Build history of the part. All positions in model axes, mm. A direction names the side the tool comes from. Give positions to 0.01 mm unless a question says otherwise; leave off trailing zeros. Loops run counter-clockwise (first coordinate to the right, second up) from the corner with the lowest first, then second, coordinate; pieces in that order, holes last. Notation, with made-up numbers: (49, 69.25) -> (99, 69.25) arc R20 ccw to (99, 95.25) -> close; hole circle Ø1 at (5, -6). An arc over 180 degrees is marked (long way). Answer in a Markdown table with one row per item. Add a question column.
from build123d import *

# Parameters (mm, degrees)
F1_DEPTH = 76.2
F2_R     = 38.1


# Not quite as in the source:
# - ends of sketch curves that miss each other by under 0.0002 mm in the source are joined


with BuildPart() as f1:
    # F0 (on Top) → F1 (new body, symmetric)
    with BuildSketch(Plane.XY):
        Polygon((21.6444802228, 76.2), (-21.6444802228, 76.2), (-21.6444802228, -50.8097953513), (-55.2607951227, -50.8097953513), (-54.5555197772, -76.2), (-21.6444802228, -76.2), (21.6444802228, -76.2), align=None)
    extrude(amount=F1_DEPTH, both=True)

    # F2
    f2_edges = [f1.edges().sort_by_distance(p)[0] for p in [
        (0, 76.2, -76.2),
        (0, 76.2, 76.2),
    ]]
    fillet(f2_edges, radius=F2_R)


solid = f1.part
(1) Saw through at C-C, the plane y = 23. List the corners of the cut face in (x, z).
(2) Flat gauge pins, fed straight in: pin 1 Ø17 at (x, z) = (-41, -1.5) entering from +Y; pin 2 Ø5 at (y, z) = (45.5, 15) entering from -X. Where does each tip first touch, or does it go through?
(3) Wall check: line 1 along Y through (x, z) = (-30, 32); line 2 along X through (y, z) = (-41.5, 58); line 3 along Z through (x, y) = (-11, 41.5). Give the ranges that are in metal, low to high. Write a range as from..to.
(4) 3-axis set-ups, long thin cutter, end or side, ignore diameter. For faces 4 (the flat face through (-21.644, 14, 1)), 5 (the flat face through (-9, -31, 76.2)): which of +Z, -Z, +X, -X, +Y, -Y reach the whole face in a straight line?
(5) Saw through at B-B, the plane x = -34. List the corners of the cut face in (y, z), then the cut area to 3 significant figures.
(6) Saw through at A-A, the plane z = -1. List the corners of the cut face in (x, y), then the cut area to 3 significant figures.
(7) Two-plate mould, pull along Z, no slides. Class faces 1 (the flat face through (-9, -31, -76.2)), 2 (the flat face through (-17, -76.2, 1)), 3 (the cylindrical face through (-0.3, 65.34, 64.74)): released by +Z, released by -Z, zero draft, split by the parting line, or undercut.
(8) Saw through at D-D, the plane x = 13.5. List the corners of the cut face in (y, z), then the cut area to 3 significant figures.
Worked answers:
| question | item | result |
|---|---|---|
| 1 | outline | (-21.64, -76.2) -> (21.64, -76.2) -> (21.64, 76.2) -> (-21.64, 76.2) -> close |
| 2 | pin 1 | y = -50.81 |
| 2 | pin 2 | x = -21.64 |
| 3 | line 1 | -76.2..-50.81 |
| 3 | line 2 | -21.64..21.64 |
| 3 | line 3 | -76.05..76.05 |
| 4 | face 4 | +Z, -Z, -X, +Y |
| 4 | face 5 | +Z, +X, -X, +Y, -Y |
| 5 | outline | (-76.2, -76.2) -> (-50.81, -76.2) -> (-50.81, 76.2) -> (-76.2, 76.2) -> close |
| 5 | area | 3,870 mm^2 |
| 6 | outline | (-55.26, -50.81) -> (-54.56, -76.2) -> (21.64, -76.2) -> (21.64, 76.2) -> (-21.64, 76.2) -> (-21.64, -50.81) -> close |
| 6 | area | 7,440 mm^2 |
| 7 | face 1 | released by -Z |
| 7 | face 2 | zero draft |
| 7 | face 3 | released by +Z |
| 8 | outline | (-76.2, -76.2) -> (38.1, -76.2) arc R38.1 ccw to (76.2, -38.1) -> (76.2, 38.1) arc R38.1 ccw to (38.1, 76.2) -> (-76.2, 76.2) -> close |
| 8 | area | 22,600 mm^2 |
